Part model, mm, in its own coordinate system. A direction names the side the tool comes from. Round coordinates to 2 decimals unless told otherwise and drop trailing zeros. Order: outer loops, then holes, each group sorted by start corner. A loop starts at its lowest first (then second) coordinate and runs counter-clockwise, first axis right, second up. Notation, with made-up numbers: (-4.5, 85.5) -> (28.5, 85.5) arc R21 ccw to (28.5, 117.5) -> close; hole circle Ø6 at (-17, 72.5). An arc over 180 degrees is marked (long way). Answer as a JSON object with one key per item and string values. Group by question number.
```python
from build123d import *

# Parameters (mm, degrees)
F0_W     = 500
F0_H     = 120
F1_DEPTH = 500
F2_T     = -20
F3_W     = 460
F3_H     = 460
F4_DEPTH = 45


with BuildPart() as f1:
    # F0 (on Front) → F1 (new body)
    with BuildSketch(Plane.XZ):
        with Locations((250, 60)):
            Rectangle(F0_W, F0_H)
    extrude(amount=-F1_DEPTH)

    # F2
    f2_openings = [f1.faces().sort_by_distance(p)[0] for p in [
        (250, 250, 120),
    ]]
    offset(amount=F2_T, openings=f2_openings)

    # F3 (on face) → F4 (join)
    with BuildSketch(Plane.XY.offset(20)):
        with Locations((250, 250)):
            Rectangle(F3_W, F3_H)
    extrude(amount=F4_DEPTH)


solid = f1.part
```
Q1. Which spindle directions (+Z, -Z, +X, -X, +Y, -Y) get a long thin tool onto all of the face, cutting with end or side? Do faces 4 (the flat face through (247, 20, 93)), 5 (the flat face through (247, 246, 0)). Say none if no direction does.
Q2. Wall check: line 1 (X direction, y = 26, z = 87); line 2 (Z direction, x = 215.5, y = 433.5). Give the ranges that are in metal, low to high. Write a range as [from, to].
Q3. Drop a flat-ended pin along its axis: pin 1 Ø6 at (x, y) = (359, 332) entering from +Z. Give the stop position or say it passes through.
Q4. Two-plate mould, pull along Y, no slides. Class faces 1 (the flat face through (20, 247, 92)), 2 (the flat face through (230, 490, 120)), 3 (the flat face through (247, 0, 61)): +Y half, -Y half, draft (parallel to the pull), parting line (faces both ways), or undercut.
Q5. Band-saw the part on A-A (z = 104). List the corners of the cut face in (x, y), plus the area to 3 significant figures.
Q6. Band-saw the part on B-B (x = 364.5). List the corners of the cut face in (y, z).
Completed:
{
 "1": {"face 4": "+Z", "face 5": "-Z, +X, -X, +Y, -Y"},
 "2": {"line 1": "[0, 20], [480, 500]", "line 2": "[0, 65]"},
 "3": {"pin 1": "z = 65"},
 "4": {"face 1": "undercut", "face 2": "draft", "face 3": "-Y half"},
 "5": {"outline": "(0, 0) -> (500, 0) -> (500, 500) -> (0, 500) -> close; hole (20, 20) -> (480, 20) -> (480, 480) -> (20, 480) -> close", "area": "38,400 mm2"},
 "6": {"outline": "(0, 0) -> (500, 0) -> (500, 120) -> (480, 120) -> (480, 65) -> (20, 65) -> (20, 120) -> (0, 120) -> close"}
}
